Geometry check sheet. Reference: the model listing, model coordinates, mm. Face numbers are marked on the shaded views. A direction names the side the tool comes from. Give positions to 0.01 mm unless a question says otherwise; leave off trailing zeros. Order: outer loops, then holes, each group sorted by start corner. A loop starts at its lowest first (then second) coordinate and runs counter-clockwise, first axis right, second up. Notation, with made-up numbers: M 32,16.25 L 89,16.25 A10 ccw 89,27.25 Z; hole C 6.25,39.25 d8. An arc over 180 degrees is marked long. Answer as a JSON object with one key per item and string values. Group by question number.
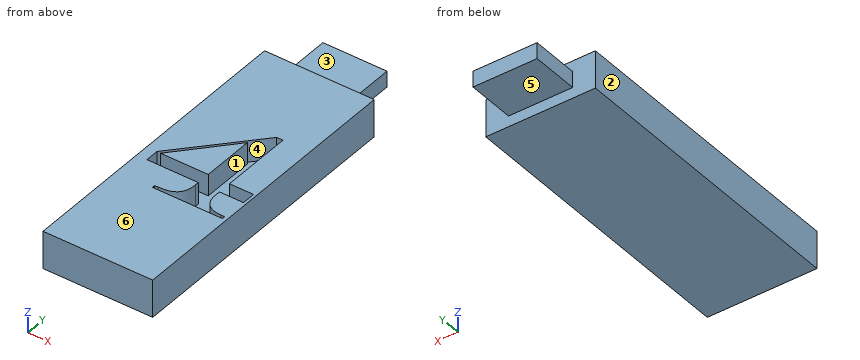
from build123d import *

# Parameters (mm, degrees)
SKETCH1_W           = 17.38
SKETCH1_H           = 47.498
BOSS_EXTRUDE1_DEPTH = 5.95
CUT_EXTRUDE1_DEPTH  = 3.41
SKETCH3_W           = 10.16
SKETCH3_H           = 2.54
BOSS_EXTRUDE2_DEPTH = 7.62


with BuildPart() as part:
    # Sketch1 → Boss-Extrude1 (new body)
    with BuildSketch(Plane.XY):
        Rectangle(SKETCH1_W, SKETCH1_H)
    extrude(amount=BOSS_EXTRUDE1_DEPTH)

    # Sketch2 → Cut-Extrude1 (cut)
    with BuildSketch(Plane.XY.offset(5.95)):
        with BuildLine():
            Line((3.438639944, 9.924455156), (4.442467735, 9.924455156))
            Line((4.442467735, 9.924455156), (4.442467735, -1.539332851))
            Line((4.442467735, -1.539332851), (8.256267, -1.539332851))
            Line((8.256267, -1.539332851), (8.256267, -3.688793102))
            Line((8.256267, -3.688793102), (4.442467735, -3.688793102))
            Line((4.442467735, -3.688793102), (4.442467735, -4.640377068))
            add(Edge.make_bspline(
                [(4.442467735, -4.640377068), (4.443669751, -4.751273799), (4.44601529, -4.967670812), (4.491573849, -5.280067729), (4.547428573, -5.576451443), (4.638679375, -5.850580816), (4.750284326, -6.109988852), (4.893045349, -6.345559529), (5.054243786, -6.56764849), (5.24539936, -6.764114691), (5.45895144, -6.939280612), (5.690437988, -7.094166195), (5.94412251, -7.21948209), (6.213330934, -7.330421399), (6.505331291, -7.411643013), (6.816896163, -7.464731494), (7.145657743, -7.505427509), (7.371717246, -7.508487842), (7.487536425, -7.510055771)],
                knots=[0, 0, 0, 0, 1.118672576, 2.182908393, 3.183164075, 4.160436979, 5.09410661, 6.029127428, 6.936133637, 7.860118871, 8.788194062, 9.721948199, 10.665788183, 11.640878679, 12.658961174, 13.718515742, 14.83110584, 16, 16, 16, 16], degree=3))
            Line((7.487536425, -7.510055771), (8.080877015, -7.510055771))
            Line((8.080877015, -7.510055771), (8.080877015, -7.987713605))
            Line((8.080877015, -7.987713605), (-2.994814002, -7.987713605))
            Line((-2.994814002, -7.987713605), (-2.994814002, -7.510055771))
            Line((-2.994814002, -7.510055771), (-2.453717238, -7.510055771))
            add(Edge.make_bspline(
                [(-2.453717238, -7.510055771), (-2.258238674, -7.505911681), (-1.884825234, -7.49799542), (-1.351318965, -7.434422338), (-0.871964817, -7.331943938), (-0.442786011, -7.18885029), (-0.068953302, -6.991569685), (0.256975704, -6.754501307), (0.523821338, -6.462132653), (0.738539375, -6.124798114), (0.904653386, -5.736728404), (1.016200957, -5.296067491), (1.08879249, -4.804482414), (1.095404798, -4.459053985), (1.0988629, -4.278401991)],
                knots=[0, 0, 0, 0, 1.266752721, 2.419817719, 3.476234114, 4.440044039, 5.341650734, 6.205967801, 7.039034094, 7.891156267, 8.786794986, 9.762669761, 10.829922107, 12, 12, 12, 12], degree=3))
            Line((1.0988629, -4.278401991), (1.0988629, -3.688793102))
            Line((1.0988629, -3.688793102), (-7.047442184, -3.688793102))
            Line((-7.047442184, -3.688793102), (-7.047442184, -1.539332851))
            Line((-7.047442184, -1.539332851), (3.438639944, 9.924455156))
        make_face()
        Polygon((1.0988629, 6.819679237), (-6.457833296, -1.565454764), (1.0988629, -1.565454764), align=None, mode=Mode.SUBTRACT)
    extrude(amount=-CUT_EXTRUDE1_DEPTH, mode=Mode.SUBTRACT)

    # Sketch3 → Boss-Extrude2 (add)
    with BuildSketch(Plane(origin=(0, 23.749, 0), x_dir=(1, 0, 0), z_dir=(0, 1, 0))):
        with Locations((0, -2.975)):
            Rectangle(SKETCH3_W, SKETCH3_H)
    extrude(amount=BOSS_EXTRUDE2_DEPTH)


solid = part.part
1. Cross-section at A-A (z = 4.8). State how many separate pieces and enclosed holes the cut face has, and give its area (3 significant figures).
2. Access from +Z, -Z, +X, -X, +Y, -Y to the whole of each face (thin tool, end or side, straight path). Record for the marked faces 4, 5 and 6.
3. Cross-section at D-D (y = 25.5). Record the cut outline in (x, z) (3 decimals), and give its area (3 significant figures).
4. Thickness scan on line 1 along Y through (x, z) = (1.75, 2.85); line 2 along Y through (x, z) = (6.25, 4.45); line 3 along X through (y, z) = (-1.5, 4). Record the ranges inside material, lowest first. Write a range as [from, to].
5. Depth check by flat-ended pin: pin 1 (3 mm diameter, centred on y = 28, z = 3.5, fed in from +X); pin 2 (1 mm diameter, centred on y = 25.5, z = 2.5, fed in from -X). Enter the tip coordinate at first touch or a pass-through.
6. Cross-section at C-C (x = -3.5). Record the cut outline in (y, z) (3 decimals).
7. Cross-section at B-B (y = 2). Record the cut outline in (x, z).
8. Release check for a two-part mould opening along X. For the marked faces 1, 2 and 3 record: released by +X, released by -X, zero draft, split by the parting line, or undercut.
Report:
{
 "1": {"separate pieces": "2", "enclosed holes": "1", "area": "731 mm2"},
 "2": {"face 4": "+Z", "face 5": "-Z, +X, -X, +Y", "face 6": "+Z, +X, -X, +Y, -Y"},
 "3": {"outline": "M -5.08,1.705 L 5.08,1.705 L 5.08,4.245 L -5.08,4.245 Z", "area": "25.8 mm2"},
 "4": {"line 1": "y = [-23.75, -7.99], [8.08, 31.37]", "line 2": "y = [-23.75, -7.99], [-7.34, -3.69], [-1.54, 23.75]", "line 3": "x = [-8.69, -7.01], [-6.4, 1.1], [4.44, 8.69]"},
 "5": {"pin 1": "stops at x = 5.08", "pin 2": "stops at x = -5.08"},
 "6": {"outline": "M -23.749,0 L 23.749,0 L 23.749,1.705 L 31.369,1.705 L 31.369,4.245 L 23.749,4.245 L 23.749,5.95 L 2.339,5.95 L 2.339,2.54 L 1.717,2.54 L 1.717,5.95 L -1.565,5.95 L -1.565,2.54 L -3.689,2.54 L -3.689,5.95 L -23.749,5.95 Z"},
 "7": {"outline": "M -8.69,0 L 8.69,0 L 8.69,5.95 L 4.44,5.95 L 4.44,2.54 L 1.1,2.54 L 1.1,5.95 L -3.24,5.95 L -3.24,2.54 L -3.81,2.54 L -3.81,5.95 L -8.69,5.95 Z"},
 "8": {"face 1": "undercut", "face 2": "released by -X", "face 3": "zero draft"}
}
